Drawing for the job (mm, zero at the part's lowest x, y, z). A direction names the side the tool comes from. Round coordinates to 2 decimals unless told otherwise and drop trailing zeros. Write each loop counter-clockwise with the first axis right and the second up, starting at its lowest first coordinate (ties: lowest second). Pieces come first, ordered by that corner, then holes. Notation, with made-up numbers: M 5.5,-39.5 L 24.5,-39.5 A30 ccw 24.5,-13.5 Z; hole C 37,5.5 d4. An arc over 180 degrees is marked long. Use a Markdown table: item, result. Add a question column.
1) Slice it at D-D on x = 15. Write the cut outline in (y, z).
2) Which spindle directions (+Z, -Z, +X, -X, +Y, -Y) get a long thin tool onto all of the face, cutting with end or side? Do the marked faces 1, 2, 3, 4 and 5. Say none if no direction does.
3) Slice it at C-C on x = 55.5. Write the cut outline in (y, z).
4) Two-plate mould, pull along Z, no slides. Class the marked faces 6, 7, 8 and 9: released by +Z, released by -Z, zero draft, split by the parting line, or undercut.
5) Slice it at B-B on z = 15. Write the cut outline in (x, y), plus the area to 3 significant figures.
6) Wall check: probe 1 along Y at (x, z) = (32, 10); probe 2 along X at (y, z) = (24, 9.5); probe 3 along X at (y, z) = (12, 29). Give the ranges that are in metal, low to high.
7) Drop flat-ended pins along their axis: P1, Ø21, axis at x = 8.5, z = 37.5, coming from the -Y side; P2, Ø2, axis at x = 2.5, y = 14.5, coming from the +Z side; P3, Ø7, axis at y = 22.5, z = 4.5, coming from the +X side; P4, Ø1.5, axis at y = 8.5, z = 20, coming from the -X side. Give the stop position or say it passes through.
8) Slice it at A-A on y = 19. Write the cut outline in (x, z) (1 decimal).
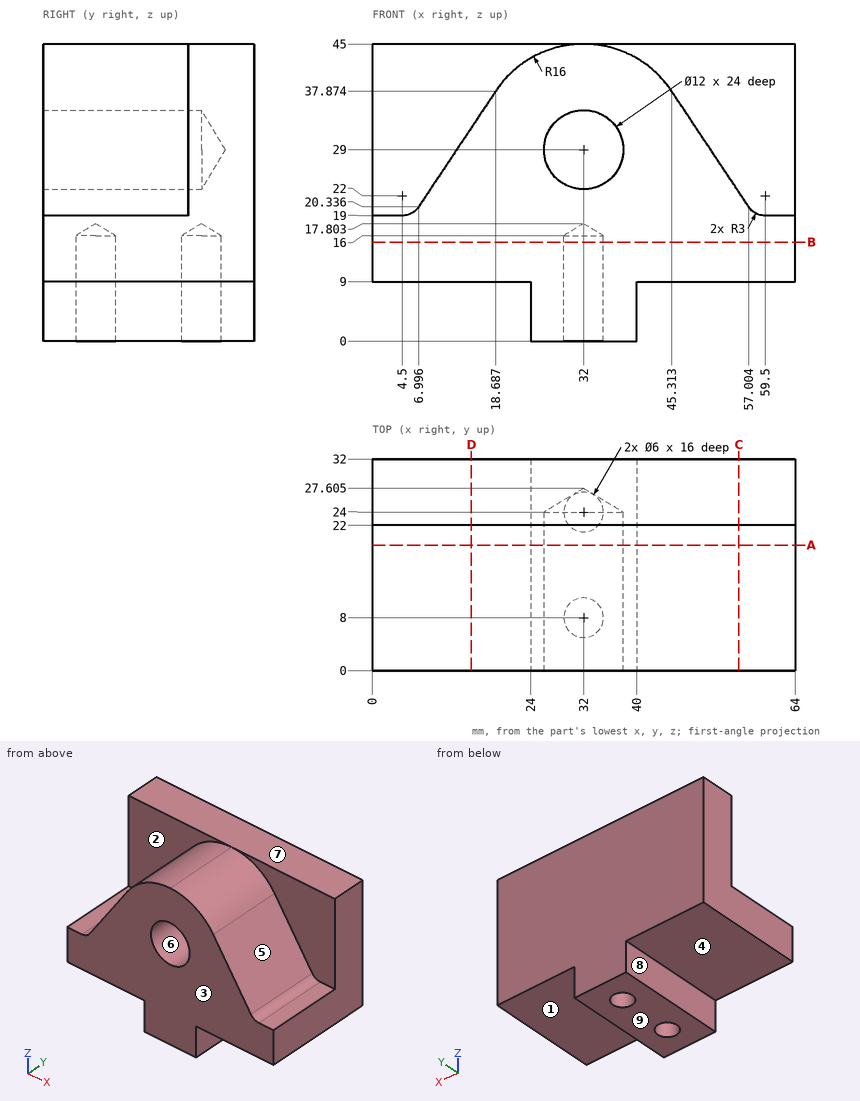
Entries:
| question | item | result |
|---|---|---|
| 1 | outline | M 0,9 L 32,9 L 32,45 L 22,45 L 22,32.34 L 0,32.34 Z |
| 2 | face 1 | -Z, +X, +Y, -Y |
| 2 | face 2 | +Z, -X, -Y |
| 2 | face 3 | +Z, -Z, +X, -X, -Y |
| 2 | face 4 | -Z, -X, +Y, -Y |
| 2 | face 5 | +Z, +X, -Y |
| 3 | outline | M 0,9 L 32,9 L 32,45 L 22,45 L 22,22.59 L 0,22.59 Z |
| 4 | face 6 | undercut |
| 4 | face 7 | released by +Z |
| 4 | face 8 | zero draft |
| 4 | face 9 | released by -Z |
| 5 | outline | M 0,0 L 64,0 L 64,32 L 0,32 Z; hole C 32,8 d6; hole C 32,24 d6 |
| 5 | area | 1,990 mm^2 |
| 6 | probe 1 | y = 0 to 5, 11 to 21, 27 to 32 |
| 6 | probe 2 | x = 0 to 29, 35 to 64 |
| 6 | probe 3 | x = 12.77 to 26, 38 to 51.23 |
| 7 | P1 | stops at y = 0 |
| 7 | P2 | stops at z = 19 |
| 7 | P3 | stops at x = 40 |
| 7 | P4 | stops at x = 5.7 |
| 8 | outline | M 0,9 L 24,9 L 24,0 L 40,0 L 40,9 L 64,9 L 64,19 L 59.5,19 A3 cw 57,20.3 L 45.3,37.9 A16 ccw 18.7,37.9 L 7,20.3 A3 cw 4.5,19 L 0,19 Z; hole C 32,29 d12 |
